from build123d import *

# Parameters (mm, degrees)
BOSS_EXTRUDE1_DEPTH   = 3.175
SKETCH5_R             = 7.9375
CUT_EXTRUDE2_DEPTH    = 163.67034341
F_8_CLEARANCE_HOLE2_D = 4.3053
SKETCH8_R             = 14.2875
CUT_EXTRUDE3_DEPTH    = 163.67034341


with BuildPart() as part:
    # Sketch1 → Boss-Extrude1 (new body)
    with BuildSketch(Plane.XY):
        Polygon((0, 101.6), (-101.6, 69.85), (-101.6, 0), (0, 0), (127, 0), (127, 69.85), (25.4, 101.6), align=None)
    extrude(amount=BOSS_EXTRUDE1_DEPTH)

    # Sketch5 → Cut-Extrude2 (cut, through all)
    with BuildSketch(Plane(origin=(0, 0, 0), x_dir=(-1, 0, 0), z_dir=(0, 0, -1))):
        with Locations((80.6, 47.625)):
            Circle(SKETCH5_R)
    extrude(amount=-CUT_EXTRUDE2_DEPTH, mode=Mode.SUBTRACT)

    # #8 Clearance Hole2 (through all)
    with Locations(Plane(origin=(0, 0, 0), x_dir=(-1, 0, 0), z_dir=(0, 0, -1))):
        with Locations((80.6, 47.625), (98.33, 29.895), (62.87, 65.355), (62.87, 29.895), (98.33, 65.355)):
            Hole(F_8_CLEARANCE_HOLE2_D / 2)

    # Sketch8 → Cut-Extrude3 (cut, through all)
    with BuildSketch(Plane(origin=(0, 0, 0), x_dir=(-1, 0, 0), z_dir=(0, 0, -1))):
        with Locations((30.607, 56.643866392)):
            Circle(SKETCH8_R)
    extrude(amount=-CUT_EXTRUDE3_DEPTH, mode=Mode.SUBTRACT)


solid = part.part
Check sheet for the modelled part. Datum: model origin and axes. Units: mm. Round coordinates to 2 decimals unless told otherwise and drop trailing zeros. Loops run counter-clockwise (first coordinate to the right, second up) from the corner with the lowest first, then second, coordinate; pieces in that order, holes last. Notation, with made-up numbers: M 63.25,86 L 79.25,86 A19 ccw 79.25,103 Z; hole C 33.5,71 d6. An arc over 180 degrees is marked long. One line per item, written item: value.
(1) Release check for a two-part mould opening along X. For faces 1 (the face through (-50.089, 85.947, 1.565)), 2 (the face through (-28.75, 70.81, 1.57)), 3 (the face through (11, 40, 3.175)) record: +X half, -X half, draft (parallel to the pull), parting line (faces both ways), or undercut.
Computed values:
face 1: -X half
face 2: undercut
face 3: draft
(2) Depth check by flat-ended pin: pin 1 Ø1 at (x, z) = (-27, 0.5) entering from +Y. Enter the tip coordinate at first touch or a pass-through.
Computed values:
pin 1: stops at y = 93.32
(3) Sectioned sample at C-C, the plane y = 81. Record the cut outline in (x, z) (3 decimals).
Computed values:
outline: M -65.92,0 L 91.32,0 L 91.32,3.175 L -65.92,3.175 Z
(4) Sectioned sample at A-A, the plane z = 2.5. Count the separate pieces of the cut face and the enclosed holes in it, then the cut area to 3 significant figures.
Computed values:
separate pieces: 1
enclosed holes: 6
area: 19,100 mm^2
(5) Sectioned sample at B-B, the plane x = -98.33. Record the cut outline in (y, z) (3 decimals), then the cut area to 3 significant figures.
Computed values:
outline: M 0,0 L 27.742,0 L 27.742,3.175 L 0,3.175 Z; M 32.048,0 L 63.202,0 L 63.202,3.175 L 32.048,3.175 Z; M 67.508,0 L 70.872,0 L 70.872,3.175 L 67.508,3.175 Z
area: 198 mm^2
(6) Thickness scan on line 1 (X direction, y = 29.5, z = 1.7); line 2 (X direction, y = 51, z = 0.75); line 3 (X direction, y = 57, z = 2.15). Record the ranges inside material, lowest first.
Computed values:
line 1: x = -101.6 to -100.45, -96.21 to -64.99, -60.75 to 127
line 2: x = -101.6 to -87.78, -73.42 to -43.73, -17.48 to 127
line 3: x = -101.6 to -44.89, -16.32 to 127
(7) Sectioned sample at D-D, the plane x = -62.87. Record the cut outline in (y, z) (3 decimals).
Computed values:
outline: M 0,0 L 27.742,0 L 27.742,3.175 L 0,3.175 Z; M 32.048,0 L 63.202,0 L 63.202,3.175 L 32.048,3.175 Z; M 67.508,0 L 81.953,0 L 81.953,3.175 L 67.508,3.175 Z
